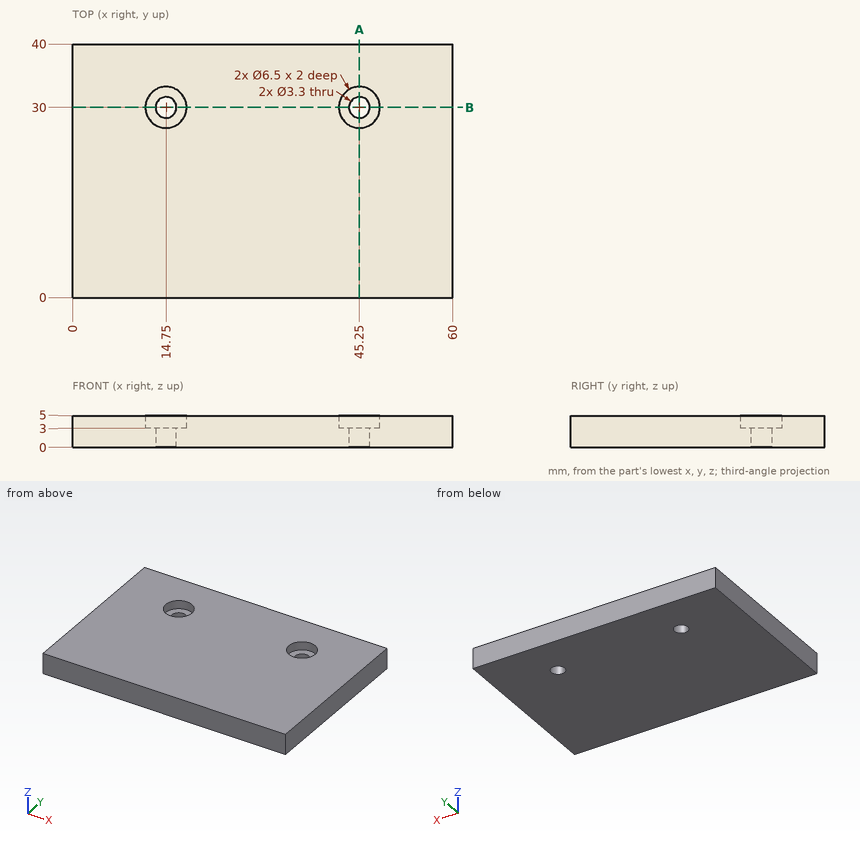
Source: three-view drawing plus pictorial views. Frame: mm from the lowest corner of the part. Give positions to 0.01 mm unless a question says otherwise; leave off trailing zeros. Write each loop counter-clockwise with the first axis right and the second up, starting at its lowest first coordinate (ties: lowest second). Pieces come first, ordered by that corner, then holes. Notation, with made-up numbers: (-27, 76) - (-21, 76) arc R16 cw to (-21, 87) - close; hole circle Ø3 at (71.5, 81). An arc over 180 degrees is marked (long way). Write item = value, one per line. Start each with the question number.
Q1. Cut plane B-B, the plane y = 30. Return loops of the section in (x, z), then the cut area to 3 significant figures.
Q2. Material intervals for probe 1 along Y at (x, z) = (45.25, 3.6); probe 2 along Y at (x, z) = (45.25, 1.45); probe 3 along Z at (x, y) = (45, 32.5), sorted ascending.
Q3. Pin query (flat end, axial travel): pin 1 Ø6 at (x, y) = (14.75, 30) entering from +Z; pin 2 Ø5 at (x, y) = (17.5, 18) entering from -Z. Return the tip coordinate at first contact, or that it passes through.
Q4. Cut plane A-A, the plane x = 45.25. Return loops of the section in (y, z), then the cut area to 3 significant figures.
Computed values:
q1.outline = (0, 0) - (13.1, 0) - (13.1, 3) - (11.5, 3) - (11.5, 5) - (0, 5) - close; (16.4, 0) - (43.6, 0) - (43.6, 3) - (42, 3) - (42, 5) - (18, 5) - (18, 3) - (16.4, 3) - close; (46.9, 0) - (60, 0) - (60, 5) - (48.5, 5) - (48.5, 3) - (46.9, 3) - close
q1.area = 254 mm²
q2.probe_1 = 0 to 26.75, 33.25 to 40
q2.probe_2 = 0 to 28.35, 31.65 to 40
q2.probe_3 = 0 to 3
q3.pin_1 = 3
q3.pin_2 = 0
q4.outline = (0, 0) - (28.35, 0) - (28.35, 3) - (26.75, 3) - (26.75, 5) - (0, 5) - close; (31.65, 0) - (40, 0) - (40, 5) - (33.25, 5) - (33.25, 3) - (31.65, 3) - close
q4.area = 177 mm²
